Could you check a few things on this model? Use its own coordinates, in mm. Face numbers are marked on the shaded views. A direction names the side the tool comes from. Give positions to 0.01 mm unless a question says otherwise; leave off trailing zeros. Write each loop counter-clockwise with the first axis right and the second up, starting at its lowest first coordinate (ties: lowest second). Pieces come first, ordered by that corner, then holes. Notation, with made-up numbers: (34, -32.5) -> (66, -32.5) arc R15 cw to (66, -8.5) -> close; hole circle Ø5 at (19, -27). An arc over 180 degrees is marked (long way). Write item = value, one per line. Start each with the question number.
Autodesk Inventor part; units mm, degrees
ref_plane "YZ Plane" through (0, 0, 0) normal (1, 0, 0) x (0, 1, 0)
ref_plane "XZ Plane" through (0, 0, 0) normal (0, 1, 0) x (-1, 0, 0)
ref_plane "XY Plane" through (0, 0, 0) normal (0, 0, 1) x (1, 0, 0)
sketch "Sketch1" plane through (0, 0, 0) normal (0, 1, 0) x (-1, 0, 0)
  line L0 (19.5703, 29.4197) -> (-40.4297, 29.4197)
  line L1 (-40.4297, 29.4197) -> (-40.4297, -15.5803)
  line L2 (-40.4297, -15.5803) -> (19.5703, -15.5803)
  line L3 (19.5703, -15.5803) -> (19.5703, 29.4197)
  point P0 (0, 0)
  dimension "d2" = 60
  dimension "d3" = 45
extrude "Extrusion1" add sketch "Sketch1" along normal blind 5
sketch "Sketch2" plane through (0, 5, 0) normal (0, 1, 0) x (1, 0, 0)
  line L0 (-19.5703, 15.5803) -> (-19.5703, -29.4197)
  line L1 (40.4297, -29.4197) -> (40.4297, 15.5803)
  line L2 (-19.5703, -29.4197) -> (40.4297, -29.4197)
  line L3 (40.4297, 15.5803) -> (-19.5703, 15.5803)
  circle A0 centre (10.4297, -6.9197) radius 3
  point P0 (0, 0)
  point P1 (13.4635, -6.9197)
extrude "Extrusion2" cut sketch "Sketch2" against normal up to next contours A0
sketch "Sketch3" plane through (0, 0, 0) normal (0, -1, 0) x (1, 0, 0)
  circle A0 centre (10.4297, 6.9197) radius 3
  circle A1 centre (10.4297, 6.9197) radius 5
  point P0 (0, 0)
  dimension "d9" = 10
extrude "Extrusion3" add sketch "Sketch3" along normal blind 10
sketch "Sketch6" plane through (0, 5, 0) normal (0, 1, 0) x (1, 0, 0)
  line L0 (-19.5703, -29.4197) -> (40.4297, -29.4197)
  line L1 (-19.5703, -29.4197) -> (-19.5703, -21.4197)
  line L2 (-19.5703, 15.5803) -> (-19.5703, -29.4197)
  line L3 (-19.5703, -21.4197) -> (40.4297, -21.4197)
  line L4 (40.4297, -29.4197) -> (40.4297, 15.5803)
  line L5 (10.4297, -29.4197) -> (10.4297, 15.5803)
  line L6 (40.4297, 15.5803) -> (-19.5703, 15.5803)
  line L7 (10.4297, -21.4197) -> (37.4297, -21.4197)
  line L8 (10.4297, -21.4197) -> (-16.5703, -21.4197)
  line L9 (-16.5703, -8.4197) -> (-9.5703, -8.4197)
  line L10 (37.4297, -21.4197) -> (37.4297, -8.4197)
  line L11 (37.4297, -8.4197) -> (30.4297, -8.4197)
  line L12 (30.4297, -8.4197) -> (30.4297, -21.4197)
  line L13 (-9.5703, -8.4197) -> (-9.5703, -21.4197)
  line L14 (-16.5703, -8.4197) -> (-16.5703, -21.4197)
  point P0 (0, 0)
  dimension "d22" = 8
  dimension "d23" = 27
  dimension "d24" = 27
  dimension "d25" = 13
  dimension "d26" = 7
  dimension "d27" = 13
  dimension "d28" = 7
extrude "Extrusion5" add sketch "Sketch6" along normal blind 20 contours L14 L9 L13 L3 | L12 L11 L10 L3
sketch "Sketch7" plane through (-16.5703, 5, 21.4197) normal (0, 0, 1) x (1, 0, 0)
  line L0 (7, 0) -> (7, 20)
  line L1 (7, 10) -> (5, 10)
  line L2 (5, 10) -> (5, 20)
  line L3 (5, 10) -> (5, 0)
  line L4 (7, 0) -> (0, 0)
  line L5 (0, 0) -> (5, 0)
  line L6 (2.5, 0) -> (2.5, 20)
  line L7 (47, 0) -> (47, 20)
  line L8 (47, 10) -> (49, 10)
  line L9 (49, 10) -> (49, 20)
  line L10 (49, 10) -> (49, 0)
  line L11 (49, 0) -> (53.9219, 0)
  line L12 (51.4609, 0) -> (51.4609, 20)
  point P0 (16.5703, -5)
  dimension "d31" = 2
  dimension "d32" = 2
sketch "Sketch8" plane through (30.4297, 5, 21.4197) normal (0, 0, 1) x (1, 0, 0)
  line L0 (2.0988, 10) -> (3.0988, 10)
  line L1 (7, 0) -> (7, 20)
  line L2 (3.0988, 12.5) -> (3.0988, 13.5)
  line L3 (0, 0) -> (0, 20)
  circle A0 centre (3.0988, 13.5) radius 1
  line L4 (3.0988, 7.5) -> (3.0988, 6.5)
  circle A1 centre (3.0988, 6.5) radius 1
  line L5 (-42.0376, 10) -> (-43.0376, 10)
  line L6 (-43.0376, 12.5) -> (-43.0376, 13.5)
  line L7 (-43.0376, 7.5) -> (-43.0376, 6.5)
  circle A2 centre (-43.0376, 13.5) radius 1
  circle A3 centre (-43.0376, 6.5) radius 1
  point P0 (-30.4297, -5)
extrude "Extrusion6" cut sketch "Sketch8" against normal blind 14
thread "Thread1"
thread "Thread2"
thread "Thread3"
thread "Thread4"
sketch "Sketch9" plane through (-19.5703, 0, 29.4197) normal (0, 0, 1) x (1, 0, 0)
  line L0 (35, 0) -> (25, 0)
  line L1 (25, -10) -> (35, -10)
  line L2 (25, 0) -> (25, -10)
  line L3 (25, -10) -> (35, -10)
  line L4 (35, -10) -> (35, 0)
  line L5 (35, 0) -> (35, -10)
  point P0 (19.5703, 0)
extrude "Extrusion7" cut sketch "Sketch9" against normal blind 40
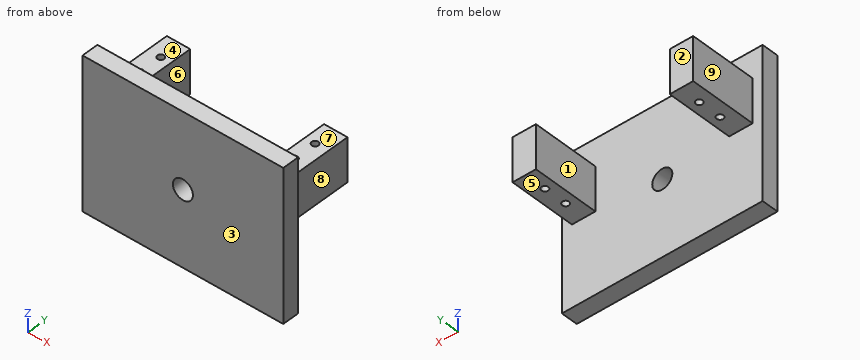
(1) Imagine slicing it at A-A (y = 14). Please give me the cut outline in (x, z), then the cut area to 3 significant figures.
(2) If I drill on line 1 along X through (y, z) = (18.5, 15); line 2 along Y through (x, z) = (18, -11.5); line 3 along Z through (x, y) = (-10, 16.5), over which ranges is the centre line in solid material (lowest first)? Write a range as from..to.
(3) On a 3-axis mill with a long thin cutter (end or side, diameter ignored), from which of +Z, -Z, +X, -X, +Y, -Y can I reach the whole of each face in a straight line? I mean the marked faces 1, 2, 3, 4 and 5. Say none if no direction works.
(4) Imagine slicing it at B-B (z = 16). Please give me the cut outline in (x, y).
(5) Imagine slicing it at C-C (z = -8). Please give me the cut outline in (x, y), then the cut area to 3 significant figures.
(6) We'd pull the mould along X, two halves only. Please class the marked faces 6, 7, 8 and 9: released by +X, released by -X, zero draft, split by the parting line, or undercut.
(7) I'm going to push flat-ended pins straight in: pin 1 (1.6 mm diameter, centred on x = 33.53, y = 11.5, fed in from +Z); pin 2 (9.5 mm diameter, centred on x = 10.43, z = 6.92, fed in from +Y); pin 3 (2.5 mm diameter, centred on x = -12.61, y = 18.5, fed in from -Z); pin 4 (6.5 mm diameter, centred on y = 18, z = 14, fed in from -X). Where does each tip first touch, or does it pass through?
Answers below:
q1.outline = (-16.57, 8.42) -> (-9.57, 8.42) -> (-9.57, 21.42) -> (-16.57, 21.42) -> close; (30.43, 8.42) -> (37.43, 8.42) -> (37.43, 21.42) -> (30.43, 21.42) -> close
q1.area = 182 mm^2
q2.line_1 = -16.57..-13.61, -11.61..-9.57, 30.43..32.53, 34.53..37.43
q2.line_2 = 0..5
q2.line_3 = 8.42..21.42
q3.face_1 = +Z, -Z, +Y
q3.face_2 = +Z, -Z, +X, -X, +Y
q3.face_3 = +Z, -Z, +X, -X, -Y
q3.face_4 = +Z, +X, -X, +Y
q3.face_5 = -Z, +X, -X, +Y
q4.outline = (-19.57, 0) -> (40.43, 0) -> (40.43, 5) -> (37.43, 5) -> (37.43, 25) -> (30.43, 25) -> (30.43, 5) -> (-9.57, 5) -> (-9.57, 25) -> (-16.57, 25) -> (-16.57, 5) -> (-19.57, 5) -> close; hole circle Ø2 at (-12.61, 11.5); hole circle Ø2 at (-12.61, 18.5); hole circle Ø2 at (33.53, 11.5); hole circle Ø2 at (33.53, 18.5)
q5.outline = (-19.57, 0) -> (40.43, 0) -> (40.43, 5) -> (-19.57, 5) -> close
q5.area = 300 mm^2
q6.face_6 = undercut
q6.face_7 = zero draft
q6.face_8 = released by +X
q6.face_9 = released by -X
q7.pin_1 = through
q7.pin_2 = 5
q7.pin_3 = 8.42
q7.pin_4 = -16.57
